Autodesk Fusion 360 part; units mm, degrees
sketch "Esboço1" plane through (0, 0, 0) normal (0, 0, 1) x (1, 0, 0)
  line L0 (0, 0) -> (28.4, 0)
  line L1 (28.4, 0) -> (28.4, 58.2)
  line L2 (28.4, 58.2) -> (0, 58.2)
  line L3 (0, 58.2) -> (0, 0)
  line L4 (-5.0078, -5.0078) -> (33.4078, -5.0078)
  line L5 (33.4078, -5.0078) -> (33.4078, 63.2078)
  line L6 (33.4078, 63.2078) -> (-5.0078, 63.2078)
  line L7 (-5.0078, 63.2078) -> (-5.0078, -5.0078)
  dimension "d1" = 28.4
  dimension "d2" = 58.2
  dimension "d3" = 5.0078
extrude "Extrusão1" add sketch "Esboço1" along normal blind 10 makes body 1
sketch "Esboço2" plane through (0, 0, 0) normal (0, 1, 0) x (-1, 0, 0)
  line L0 (-28.4, 0) -> (0, 0)
  line L1 (0, 0) -> (0, 10)
  line L2 (0, 10) -> (-28.4, 10)
  line L3 (-28.4, 10) -> (-28.4, 0)
  line L4 (-14.2, 0) -> (-17.2, 0)
  line L5 (-17.2, 0) -> (-17.2, 10)
  line L6 (-17.2, 10) -> (-14.2, 10)
  line L7 (-14.2, 10) -> (-14.2, 0)
  line L8 (-14.2, 0) -> (-11.2, 0)
  line L9 (-11.2, 0) -> (-11.2, 10)
  line L10 (-11.2, 10) -> (-14.2, 10)
  line L11 (-14.2, 10) -> (-14.2, 0)
  dimension "d6" = 3
extrude "Extrusão2" cut sketch "Esboço2" along normal blind -0.6 and the other way blind -58.8 contours L0 L2 L4 L5 L6 L7 L11 | L0 L2 L7 L8 L9 L10 L11 bodies 1
sketch "Esboço3" plane through (0, 58.8, 0) normal (0, -1, 0) x (1, 0, 0)
  line L0 (11.2, 0) -> (17.2, 0)
  line L1 (17.2, 0) -> (17.2, 10)
  line L2 (17.2, 10) -> (11.2, 10)
  line L3 (11.2, 10) -> (11.2, 0)
  line L4 (11.2, 5) -> (17.2, 5)
  line L5 (17.2, 4.9) -> (11.2, 4.9)
  line L6 (17.2, 5.1) -> (11.2, 5.1)
  line L7 (17.2, 5.1) -> (17.2, 4.9)
  line L8 (11.2, 5.1) -> (11.2, 4.9)
  dimension "d11" = 0.1
  dimension "d12" = 0.1
extrude "Extrusão4" cut sketch "Esboço3" against normal blind 0.3 contours L1 L3 L4 L5 L7 L8 | L1 L3 L4 L6 L7 L8 bodies 1
chamfer "Chanfro1" distance 1.2 distance2 0.3 2 edges at (14.2, 58.8, 5.1) (14.2, 58.8, 4.9) measured on face at (15.2, 58.8, 8.3667) measured on face at (15.2, 58.8, 3.2667) on bodies 1
sketch "Sketch5" plane through (0, 58.8, 0) normal (0, -1, 0) x (1, 0, 0)
  line L0 (0, 0) -> (12, 0)
  line L1 (12, 0) -> (12, 27)
  line L2 (12, 27) -> (0, 27)
  line L3 (0, 27) -> (0, 0)
  line L4 (9, 3) -> (3, 3)
  line L5 (3, 3) -> (3, 24)
  line L6 (3, 24) -> (9, 24)
  line L7 (9, 24) -> (9, 3)
  line L8 (9, 3) -> (3, 24) construction
  line L9 (3, 3) -> (9, 24) construction
  point P0 (6, 13.5)
  dimension "d25" = 12
  dimension "d26" = 27
  dimension "d27" = 6
  dimension "d28" = 21
extrude "Extrude6" add sketch "Sketch5" along normal blind 5 separate body makes body 2
sketch "Esboço4" plane through (0, -0.6, 0) normal (0, 1, 0) x (-1, 0, 0)
  line L0 (-17.2, 0) -> (-11.2, 0)
  line L1 (-11.2, 0) -> (-11.2, 10)
  line L2 (-11.2, 10) -> (-17.2, 10)
  line L3 (-17.2, 10) -> (-17.2, 0)
  line L4 (-11.2, 4.9) -> (-17.2, 4.9)
  line L5 (-11.2, 5.1) -> (-11.2, 4.9)
  line L6 (-11.2, 5.1) -> (-17.2, 5.1)
  line L7 (-17.2, 5) -> (-11.2, 5)
  line L8 (-17.2, 5.1) -> (-17.2, 4.9)
  dimension "d19" = 0.1
  dimension "d20" = 0.1
extrude "Extrusão5" cut sketch "Esboço4" against normal blind 0.3 contours L1 L3 L4 L5 L7 L8 | L1 L3 L5 L6 L7 L8 bodies 1
chamfer "Chanfro2" distance 1.2 distance2 0.3 2 edges at (14.2, -0.6, 4.9) (14.2, -0.6, 5.1) measured on face at (15.2, -0.6, 3.2667) measured on face at (15.2, -0.6, 6.7333) on bodies 1
hidden bodies 1
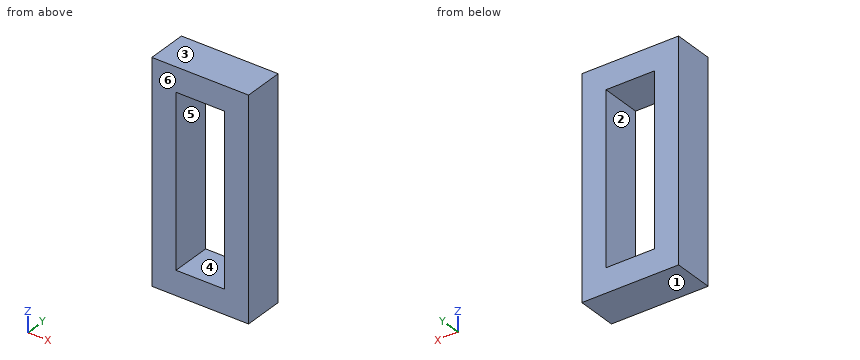
Check sheet for the modelled part. Datum: model origin and axes. Units: mm. Face numbers are marked on the shaded views. A direction names the side the tool comes from. Round coordinates to 2 decimals unless told otherwise and drop trailing zeros. Order: outer loops, then holes, each group sorted by start corner. A loop starts at its lowest first (then second) coordinate and runs counter-clockwise, first axis right, second up. Notation, with made-up numbers: M 30.25,85.25 L 87.25,85.25 A32 ccw 87.25,123.25 Z; hole C -35,87 d2. An arc over 180 degrees is marked long. One line per item, written item: value. Start each with the question number.
1. Release check for a two-part mould opening along Z. For the marked faces 1, 2, 3 and 4 record: released by +Z, released by -Z, zero draft, split by the parting line, or undercut.
2. Section check C-C on y = 57.75. Enter the section's corners in (x, z).
3. Section check B-B on z = 5. Enter the section's corners in (x, y), and give its area (3 significant figures).
4. Access from +Z, -Z, +X, -X, +Y, -Y to the whole of each face (thin tool, end or side, straight path). Record for the marked faces 5 and 6.
5. Section check A-A on x = 5. Enter the section's corners in (y, z).
6. Scan lines: line 1 along X through (y, z) = (56.25, 3.75); line 2 along Z through (x, y) = (5.75, 56.65). Record each from-to range of solid material in increasing order.
Results found:
1. face 1: released by -Z
1. face 2: undercut
1. face 3: released by +Z
1. face 4: undercut
2. outline: M 0,0 L 12,0 L 12,27 L 0,27 Z; hole M 3,3 L 9,3 L 9,24 L 3,24 Z
3. outline: M 0,53.8 L 3,53.8 L 3,58.8 L 0,58.8 Z; M 9,53.8 L 12,53.8 L 12,58.8 L 9,58.8 Z
3. area: 30.0 mm^2
4. face 5: +Y, -Y
4. face 6: +Z, -Z, +X, -X, -Y
5. outline: M 53.8,0 L 58.8,0 L 58.8,3 L 53.8,3 Z; M 53.8,24 L 58.8,24 L 58.8,27 L 53.8,27 Z
6. line 1: 0 to 3, 9 to 12
6. line 2: 0 to 3, 24 to 27
